Input: part model. Units: mm. Frame: model coordinates. A direction names the side the tool comes from. Coordinates: 2 decimals unless noted, no trailing zeros. Loops run counter-clockwise (first coordinate to the right, second up) from the corner with the lowest first, then second, coordinate; pieces in that order, holes last. Notation, with made-up numbers: M 74.25,87.25 L 86.25,87.25 A32 ccw 86.25,115.25 Z; hole C 0,1.25 d1. An arc over 180 degrees is marked long. Use a Markdown table: item, result. Add a question column.
1. Section D-D on z = -10. Output: boundary loops of the cut face in (x, y), then the cut area to 3 significant figures.
2. Section B-B on z = 12. Output: boundary loops of the cut face in (x, y).
3. Pin query (flat end, axial travel): pin 1 (5 mm diameter, centred on x = -44.5, z = -19.5, fed in from -Y); pin 2 (1.2 mm diameter, centred on x = -8, z = 4, fed in from +Y); pin 3 (3 mm diameter, centred on y = 2.5, z = 6.5, fed in from -X); pin 4 (5 mm diameter, centred on y = 1.5, z = -38, fed in from +X). Return the tip coordinate at first contact, or that it passes through.
4. Draft query along Z for faces 3 (the cylindrical face through (7.509, 7.536, 23.846)), 4 (the flat face through (-13, 0, -1)), 5 (the cylindrical face through (9.69, 2.01, 30.76)), 6 (the cylindrical face through (-3.905, 6.185, -0.867)). Return one class per face: +Z half, -Z half, draft (parallel to the pull), parting line (faces both ways), or undercut.
5. Set-up query: faces 1 (the flat face through (-19, 3, 17)), 2 (the flat face through (0, 12.2, 5)). Return all of +Z, -Z, +X, -X, +Y, -Y with unobstructed straight access to the full face (end or side cutting, diameter ignored); none if empty.
6. Line query: L1, parallel to X at y = 1.65, z = 0; L2, parallel to X at y = 11.45, z = 5; L3, parallel to Y at x = -38, z = 8.5. Output: solid intervals per line, ascending. Write a range as [from, to].
7. Section C-C on y = 8.5. Output: boundary loops of the cut face in (x, z), then the cut area to 3 significant figures.
8. Section A-A on x = -41. Output: boundary loops of the cut face in (y, z).
```python
from build123d import *

# Parameters (mm, degrees)
SKETCH1_R           = 63.5
SKETCH1_R_2         = 1.05
BOSS_EXTRUDE1_DEPTH = 3
SKETCH2_R           = 45.25
SKETCH2_R_2         = 32.25
CUT_EXTRUDE1_DEPTH  = 2
SKETCH4_R           = 25
BOSS_EXTRUDE2_DEPTH = 9.2
SKETCH5_R           = 2
CUT_EXTRUDE2_DEPTH  = 2
SKETCH6_R           = 4
CUT_EXTRUDE3_DEPTH  = 91.627479276


with BuildPart() as part:
    # Sketch1 → Boss-Extrude1 (new body)
    with BuildSketch(Plane(origin=(0, 0, 0), x_dir=(1, 0, 0), z_dir=(0, 1, 0))):
        with Locations(Location((0, 0, 0), (0, 0, 270))):
            Circle(SKETCH1_R)
        with Locations(Location((0, 61.25, 0), (0, 0, 270))):
            Circle(SKETCH1_R_2, mode=Mode.SUBTRACT)
        with Locations(Location((61.25, 0, 0), (0, 0, 270))):
            Circle(SKETCH1_R_2, mode=Mode.SUBTRACT)
        with Locations(Location((0, -61.25, 0), (0, 0, 270))):
            Circle(SKETCH1_R_2, mode=Mode.SUBTRACT)
        with Locations(Location((-61.25, 0, 0), (0, 0, 270))):
            Circle(SKETCH1_R_2, mode=Mode.SUBTRACT)
    extrude(amount=BOSS_EXTRUDE1_DEPTH)

    # Sketch2 → Cut-Extrude1 (cut)
    with BuildSketch(Plane(origin=(0, 3, 0), x_dir=(1, 0, 0), z_dir=(0, 1, 0))):
        with Locations(Location((0, 0, 0), (0, 0, 270))):
            Circle(SKETCH2_R)
        with Locations(Location((0, 0, 0), (0, 0, 270))):
            Circle(SKETCH2_R_2, mode=Mode.SUBTRACT)
    extrude(amount=-CUT_EXTRUDE1_DEPTH, mode=Mode.SUBTRACT)

    # Sketch4 → Boss-Extrude2 (add)
    with BuildSketch(Plane(origin=(0, 3, 0), x_dir=(1, 0, 0), z_dir=(0, 1, 0))):
        with Locations(Location((0, 0, 0), (0, 0, 270))):
            Circle(SKETCH4_R)
    extrude(amount=BOSS_EXTRUDE2_DEPTH)

    # Sketch5 → Cut-Extrude2 (cut)
    with BuildSketch(Plane(origin=(0, 12.2, 0), x_dir=(1, 0, 0), z_dir=(0, 1, 0))):
        with Locations(Location((0, 10, 0), (0, 0, 270))):
            Circle(SKETCH5_R)
        with Locations(Location((8.660254038, -5, 0), (0, 0, 270))):
            Circle(SKETCH5_R)
        with Locations(Location((-8.660254038, -5, 0), (0, 0, 270))):
            Circle(SKETCH5_R)
    extrude(amount=-CUT_EXTRUDE2_DEPTH, mode=Mode.SUBTRACT)

    # Sketch6 → Cut-Extrude3 (cut, through all)
    with BuildSketch(Plane(origin=(0, 12.2, 0), x_dir=(1, 0, 0), z_dir=(0, 1, 0))):
        with Locations(Location((0, 0, 0), (0, 0, 270))):
            Circle(SKETCH6_R)
    extrude(amount=-CUT_EXTRUDE3_DEPTH, mode=Mode.SUBTRACT)


solid = part.part
```
Answers below:
| question | item | result |
|---|---|---|
| 1 | outline | M -62.71,0 L 62.71,0 L 62.71,3 L 44.13,3 L 44.13,1 L 30.66,1 L 30.66,3 L 22.91,3 L 22.91,12.2 L 2,12.2 L 2,10.2 L -2,10.2 L -2,12.2 L -22.91,12.2 L -22.91,3 L -30.66,3 L -30.66,1 L -44.13,1 L -44.13,3 L -62.71,3 Z |
| 1 | area | 736 mm² |
| 2 | outline | M -62.36,0 L 62.36,0 L 62.36,3 L 43.63,3 L 43.63,1 L 29.93,1 L 29.93,3 L 21.93,3 L 21.93,12.2 L -21.93,12.2 L -21.93,3 L -29.93,3 L -29.93,1 L -43.63,1 L -43.63,3 L -62.36,3 Z |
| 3 | pin 1 | stops at y = 0 |
| 3 | pin 2 | stops at y = 10.2 |
| 3 | pin 3 | stops at x = -63.3 |
| 3 | pin 4 | stops at x = 52.65 |
| 4 | face 3 | parting line |
| 4 | face 4 | draft |
| 4 | face 5 | undercut |
| 4 | face 6 | undercut |
| 5 | face 1 | +Y |
| 5 | face 2 | +Z, -Z, +X, -X, +Y |
| 6 | L1 | x = [-63.5, -62.3], [-60.2, -45.25], [-32.25, -4], [4, 32.25], [45.25, 60.2], [62.3, 63.5] |
| 6 | L2 | x = [-24.49, -10.66], [-6.66, 6.66], [10.66, 24.49] |
| 6 | L3 | y = [0, 1] |
| 7 | outline | C 0,0 d50; hole C 0,0 d8 |
| 7 | area | 1,910 mm² |
| 8 | outline | M 0,-48.49 L 3,-48.49 L 3,-19.15 L 1,-19.15 L 1,19.15 L 3,19.15 L 3,48.49 L 0,48.49 Z |
